Part model, mm, in its own coordinate system. A direction names the side the tool comes from. Coordinates: 2 decimals unless noted, no trailing zeros. Write each loop counter-clockwise with the first axis right and the second up, starting at its lowest first coordinate (ties: lowest second). Pieces come first, ordered by that corner, then holes. Notation, with made-up numbers: (-17, 38) -> (30, 38) arc R5 cw to (30, 45) -> close; hole circle Ø4 at (89, 74). An arc over 180 degrees is marked (long way). Write item = value, one per line. Start each with the question number.
Q1. Tool access for faces 1 (the flat face through (-25, -20, 6)), 2 (the cylindrical face through (15, -29, 45)), 3 (the flat face through (23, -22, 5)): list every direction of +Z, -Z, +X, -X, +Y, -Y with a clear straight run to the whole face (end or side of a thin tool).
Q2. Band-saw the part on B-B, the plane z = 16.5. List the corners of the cut face in (x, y), plus the area to 3 significant figures.
Q3. Band-saw the part on D-D, the plane x = 15.5. List the corners of the cut face in (y, z).
Q4. Band-saw the part on A-A, the plane y = 0. List the corners of the cut face in (x, z), plus the area to 3 significant figures.
Q5. Probe line 1 (Y direction, x = -15.5, z = -1.5); line 2 (X direction, y = -15, z = -2); line 3 (Z direction, x = 20.5, y = 8). List the from-to ranges inside material, lowest first.
Q6. Pull direction Z, two halves, no side cores. Call faces 4 (the flat face through (-17, -29, 28)), 5 (the flat face through (-5.2, -10.4, -3)), 6 (the flat face through (25, -20, 6)): released by +Z, released by -Z, zero draft, split by the parting line, or undercut.
Q7. Pin check, flat tips, straight feed: P1, Ø10, axis at x = 7, y = -19.5, coming from the +Z side; P2, Ø2, axis at x = -16.5, z = 39.5, coming from the +Y side. Stop position of each tip, or through.
Q8. Band-saw the part on C-C, the plane x = -9. List the corners of the cut face in (y, z).
from build123d import *

# Parameters (mm, degrees)
SKETCH_1_R      = 11.05
SKETCH_1_R_2    = 1.75
EXTRUDE_1_DEPTH = 3
EXTRUDE_2_DEPTH = 3
RIB_1_REACH     = 79.859
SKETCH_3_WALL_W = 181.571414162
SKETCH_3_WALL_H = 2
FILLET_1_R      = 2


with BuildPart() as part:
    # 草图1 → 凸台-拉伸1 (new body)
    with BuildSketch(Plane.XY):
        Polygon((-20, 21), (20, 21), (25, 16), (25, -28), (-25, -28), (-25, 16), align=None)
        Circle(SKETCH_1_R, mode=Mode.SUBTRACT)
        with Locations((15.5, 15.5)):
            Circle(SKETCH_1_R_2, mode=Mode.SUBTRACT)
        with Locations((15.5, -15.5)):
            Circle(SKETCH_1_R_2, mode=Mode.SUBTRACT)
        with Locations(Location((-15.5, -15.5, 0), (0, 0, 180))):
            Circle(SKETCH_1_R_2, mode=Mode.SUBTRACT)
        with Locations(Location((-15.5, 15.5, 0), (0, 0, 180))):
            Circle(SKETCH_1_R_2, mode=Mode.SUBTRACT)
    extrude(amount=-EXTRUDE_1_DEPTH)

    # 草图2 → 凸台-拉伸2 (add)
    with BuildSketch(Plane.XZ.offset(28)):
        Polygon((-25, -3), (-25, 46), (-20, 51), (20, 51), (25, 46), (25, -3), align=None)
        with BuildLine():
            Line((-13, 43), (-13, 13))
            ThreePointArc((-13, 13), (-15, 11), (-17, 13))
            Line((-17, 13), (-17, 43))
            ThreePointArc((-17, 43), (-15, 45), (-13, 43))
        make_face(mode=Mode.SUBTRACT)
        with BuildLine():
            Line((13, 43), (13, 13))
            ThreePointArc((13, 13), (15, 11), (17, 13))
            Line((17, 13), (17, 43))
            ThreePointArc((17, 43), (15, 45), (13, 43))
        make_face(mode=Mode.SUBTRACT)
    extrude(amount=EXTRUDE_2_DEPTH)

    # 草图3 wall → 筋1 (add, up to next)
    with BuildSketch(Plane(origin=(-25, -18, 6.5), x_dir=(0, -0.838443616301, 0.544988350595), z_dir=(0, 0.544988350595, 0.838443616301)), mode=Mode.PRIVATE) as rib_1_sk1:
        with Locations((0, 1)):
            Rectangle(SKETCH_3_WALL_W, SKETCH_3_WALL_H)
    rib_1_tool1 = extrude(rib_1_sk1.sketch, amount=-RIB_1_REACH, mode=Mode.PRIVATE) - part.part
    rib_1 = rib_1_tool1.solids().sort_by_distance((-25, -18, 6.5))[0]
    add(rib_1)

    # 镜向1: 筋1 across plane
    add(rib_1.mirror(Plane(origin=(0, 0, 0), x_dir=(0, 0, 1), z_dir=(1, 0, 0))))

    # 圆角1
    fillet_1_edges = [part.edges().sort_by_distance(p)[0] for p in [
        (0, -28, 0),
    ]]
    fillet(fillet_1_edges, radius=FILLET_1_R)


solid = part.part
Ans:
q1.face_1 = +Z, -Z, -X, +Y, -Y
q1.face_2 = +Y, -Y
q1.face_3 = +Z, +Y
q2.outline = (-25, -31) -> (-17, -31) -> (-17, -28) -> (-25, -28) -> close; (-13, -31) -> (13, -31) -> (13, -28) -> (-13, -28) -> close; (17, -31) -> (25, -31) -> (25, -28) -> (17, -28) -> close
q2.area = 126 mm2
q3.outline = (-31, -3) -> (-17.25, -3) -> (-17.25, 0) -> (-26, 0) arc R2 cw to (-28, 2) -> (-28, 11.06) -> (-31, 11.06) -> close; (-31, 44.94) -> (-28, 44.94) -> (-28, 51) -> (-31, 51) -> close; (-13.75, -3) -> (13.75, -3) -> (13.75, 0) -> (-13.75, 0) -> close; (17.25, -3) -> (21, -3) -> (21, 0) -> (17.25, 0) -> close
q4.outline = (-25, -3) -> (-11.05, -3) -> (-11.05, 0) -> (-25, 0) -> close; (11.05, -3) -> (25, -3) -> (25, 0) -> (11.05, 0) -> close
q4.area = 83.7 mm2
q5.line_1 = -31 to -17.25, -13.75 to 13.75, 17.25 to 21
q5.line_2 = -25 to -17.18, -13.82 to 13.82, 17.18 to 25
q5.line_3 = -3 to 0
q6.face_4 = undercut
q6.face_5 = released by -Z
q6.face_6 = zero draft
q7.P1 = 0
q7.P2 = -28
q8.outline = (-31, -3) -> (-6.41, -3) -> (-6.41, 0) -> (-26, 0) arc R2 cw to (-28, 2) -> (-28, 51) -> (-31, 51) -> close; (6.41, -3) -> (21, -3) -> (21, 0) -> (6.41, 0) -> close
